Geometry: see drawing. Coordinates: mm, zero at the bounding-box minimum. A direction names the side the tool comes from. Give positions to 0.01 mm unless a question says otherwise; leave off trailing zeros. Write each loop counter-clockwise with the first axis right and the second up, starting at its lowest first coordinate (ties: lowest second). Pieces come first, ordered by that corner, then holes. Notation, with made-up numbers: (-24.75, 63.25) - (-3.75, 63.25) arc R14 cw to (-3.75, 76.25) - close; hole circle Ø8 at (66.25, 15). An arc over 180 degrees is marked (long way). Return JSON: item names as keys, results as strings.
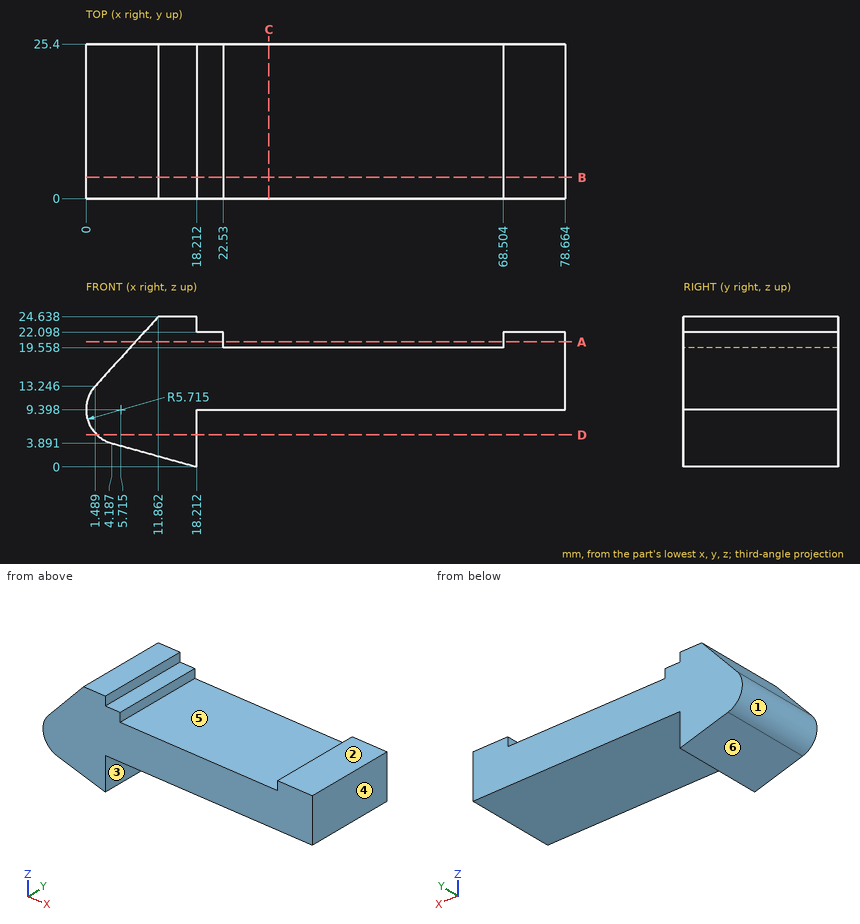
Q1. Section query C-C, the plane x = 30. Return the cut outline in (y, z).
Answer key:
{"outline": "(0, 9.4) - (25.4, 9.4) - (25.4, 19.56) - (0, 19.56) - close"}
Q2. Section query D-D, the plane z = 5.25. Return the cut outline in (x, y).
Answer key:
{"outline": "(1.78, 0) - (18.21, 0) - (18.21, 25.4) - (1.78, 25.4) - close"}
Q3. Material intervals for probe 1 along Z at (x, y) = (40, 16); probe 2 along X at (y, z) = (5.5, 20.25) (1 decimal); probe 3 along Z at (x, y) = (74.5, 24), sorted ascending. Write a range as [from, to].
Answer key:
{"probe 1": "z = [9.4, 19.56]", "probe 2": "x = [7.9, 22.5], [68.5, 78.7]", "probe 3": "z = [9.4, 22.1]"}
Q4. Section query A-A, the plane z = 20.5. Return the cut outline in (x, y) (1 decimal).
Answer key:
{"outline": "(8.1, 0) - (22.5, 0) - (22.5, 25.4) - (8.1, 25.4) - close; (68.5, 0) - (78.7, 0) - (78.7, 25.4) - (68.5, 25.4) - close"}
Q5. Set-up query: the marked faces 1, 2 and 3. Return all of +Z, -Z, +X, -X, +Y, -Y with unobstructed straight access to the full face (end or side cutting, diameter ignored); none if empty.
Answer key:
{"face 1": "-X, +Y, -Y", "face 2": "+Z, +X, +Y, -Y", "face 3": "-Z, +X, +Y, -Y"}
Q6. Mould query, pull axis X, two halves, no side actions, for the marked faces 4, 5 and 6. Classes: pulls with the +X half, pulls with the -X half, needs draft (parallel to the pull), parting line crosses it, or undercut.
Answer key:
{"face 4": "pulls with the +X half", "face 5": "undercut", "face 6": "pulls with the -X half"}
Q7. Section query B-B, the plane y = 3.5. Return the cut outline in (x, z) (1 decimal).
Answer key:
{"outline": "(1.5, 13.2) arc R5.7 ccw to (4.2, 3.9) - (18.2, 0) - (18.2, 9.4) - (78.7, 9.4) - (78.7, 22.1) - (68.5, 22.1) - (68.5, 19.6) - (22.5, 19.6) - (22.5, 22.1) - (18.2, 22.1) - (18.2, 24.6) - (11.9, 24.6) - close"}
Q8. Pin query (flat end, axial travel): P1, Ø1.3, axis at y = 9.5, z = 23, coming from the +X side; P2, Ø5, axis at y = 15, z = 20, coming from the -X side; P3, Ø12.5, axis at x = 54.5, y = 7.5, coming from the +Z side. Return the tip coordinate at first contact, or that it passes through.
Answer key:
{"P1": "stops at x = 18.21", "P2": "stops at x = 5.36", "P3": "stops at z = 19.56"}
